Geometry: see drawing. Coordinates: mm, zero at the bounding-box minimum. Coordinates: 2 decimals unless noted, no trailing zeros. Loops run counter-clockwise (first coordinate to the right, second up) from the corner with the lowest first, then second, coordinate; pieces in that order, holes last.
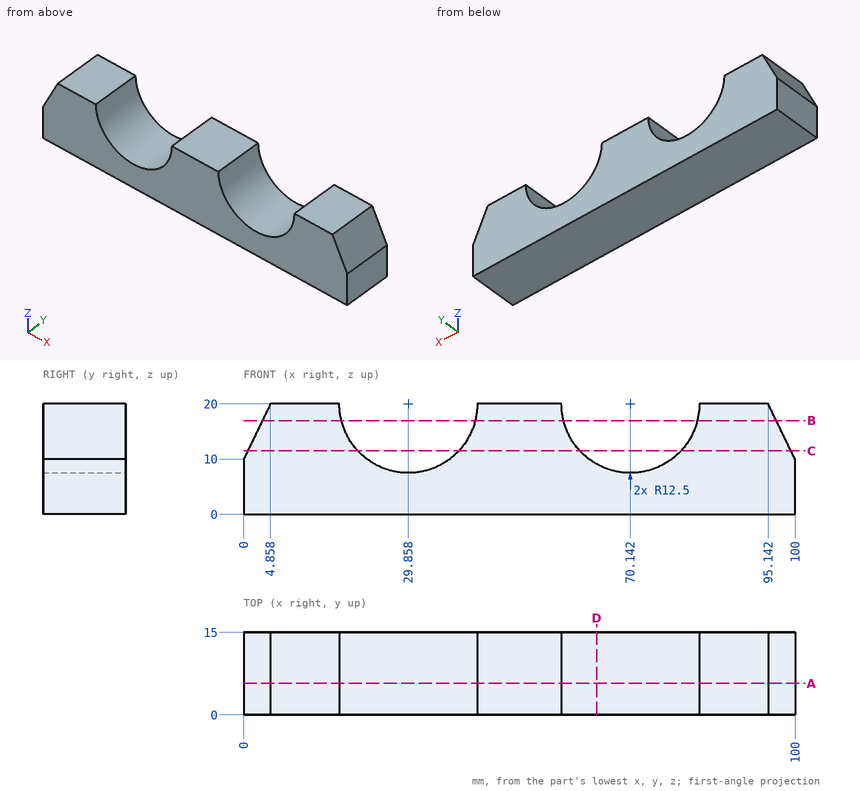
Item 1: Section query B-B (z = 17). Output: boundary loops of the cut face in (x, y).
Result:
outline: (3.4, 0) - (17.72, 0) - (17.72, 15) - (3.4, 15) - close; (41.99, 0) - (58.01, 0) - (58.01, 15) - (41.99, 15) - close; (82.28, 0) - (96.6, 0) - (96.6, 15) - (82.28, 15) - close
Item 2: Line query: L1, parallel to X at y = 5, z = 10.25 (1 decimal); L2, parallel to X at y = 14.25, z = 15.5 (1 decimal); L3, parallel to Z at x = 30, y = 7.5. Output: solid intervals per line, ascending.
Result:
L1: x = 0.1 to 22, 37.7 to 62.3, 78 to 99.9
L2: x = 2.7 to 18.2, 41.5 to 58.5, 81.8 to 97.3
L3: z = 0 to 7.5
Item 3: Section query A-A (y = 5.75). Output: boundary loops of the cut face in (x, z).
Result:
outline: (0, 0) - (100, 0) - (100, 10) - (95.14, 20) - (82.64, 20) arc R12.5 cw to (57.64, 20) - (42.36, 20) arc R12.5 cw to (17.36, 20) - (4.86, 20) - (0, 10) - close
Item 4: Section query C-C (z = 11.5). Output: boundary loops of the cut face in (x, y), then the cut area to 3 significant figures.
Result:
outline: (0.73, 0) - (20.69, 0) - (20.69, 15) - (0.73, 15) - close; (39.02, 0) - (60.98, 0) - (60.98, 15) - (39.02, 15) - close; (79.31, 0) - (99.27, 0) - (99.27, 15) - (79.31, 15) - close
area: 928 mm2
Item 5: Contact query for flat-ended pins moving along their axis: P1, Ø4, axis at x = 11, z = 9, coming from the -Y side; P2, Ø6, axis at x = 76, y = 12.5, coming from the +Z side; P3, Ø1.5, axis at x = 31.5, y = 12, coming from the +Z side. Output: stop coordinate, or through.
Result:
P1: stops at y = 0
P2: stops at z = 11.18
P3: stops at z = 7.73
Item 6: Section query D-D (x = 64). Output: boundary loops of the cut face in (y, z), then the cut area to 3 significant figures.
Result:
outline: (0, 0) - (15, 0) - (15, 9.11) - (0, 9.11) - close
area: 137 mm2
